from build123d import *

# Parameters (mm, degrees)
F1_DEPTH = 35.56
F2_W     = 27.6606
F2_H     = 23.5712
F4_DEPTH = 2.54
F7_DEPTH = 3.81
F8_DEPTH = 3.81


with BuildPart() as f1:
    # F0 (on Top) → F1 (new body)
    with BuildSketch(Plane.XY):
        Polygon((0, 12.2589374599), (0, 12.1117923089), (0, -11.4594076911), (2.54, -11.4594076911), (2.54, 12.2589374599), align=None)
    extrude(amount=F1_DEPTH)


with BuildPart() as f1_1:
    # F3: moved
    add(f1.part.moved(Location((-0.1992022446, -0.1268434648, 0))))

    # F2 (on Top) → F4 (join)
    with BuildSketch(Plane.XY):
        with Locations((16.1710977554, 0.1993488441)):
            Rectangle(F2_W, F2_H)
    extrude(amount=F4_DEPTH)

    # F5 (on face) → F7 (join)
    with BuildSketch(Plane.XZ.offset(11.5862511559)):
        Polygon((30.0013977554, 2.54), (2.3407977554, 35.56), (2.3407977554, 2.54), align=None)
    extrude(amount=-F7_DEPTH)

    # F6 (on face) → F8 (join)
    with BuildSketch(Plane(origin=(0, 12.1320939951, 0), x_dir=(-1, 0, 0), z_dir=(0, 1, 0))):
        Polygon((-2.3407977554, 35.56), (-30.0013977554, 2.54), (-2.3407977554, 2.54), align=None)
    extrude(amount=-F8_DEPTH)


solid = f1_1.part
Could you check a few things on this model? Use its own coordinates, in mm. A direction names the side the tool comes from. Coordinates: 2 decimals unless noted, no trailing zeros. Loops run counter-clockwise (first coordinate to the right, second up) from the corner with the lowest first, then second, coordinate; pieces in that order, holes last. Notation, with made-up numbers: (66, 35) -> (76, 35) arc R13 ccw to (76, 50) -> close; hole circle Ø6 at (0.5, 48). An arc over 180 degrees is marked (long way). Answer in a Markdown table with one row per item.
(1) Thinking about a two-plate mould opening in Y: for faces 4 (the face through (1, 0, 35.56)), 5 (the face through (8, 12.132, 14)), 6 (the face through (2.341, 0, 19)), which applies, released by +Y, released by -Y, zero draft, split by the parting line, or undercut?
Results found:
| item | result |
|---|---|
| face 4 | zero draft |
| face 5 | released by +Y |
| face 6 | undercut |
(2) For faces 1 (the face through (16, 0, 2.54)), 2 (the face through (16, 11.985, 1)), 3 (the face through (15, 0, 0)), which set-ups out of +Z, -Z, +X, -X, +Y, -Y let a thin tool reach every point of the face, with its end or its side?
Results found:
| item | result |
|---|---|
| face 1 | +Z, +X |
| face 2 | -Z, +X, +Y |
| face 3 | -Z, +X, -X, +Y, -Y |
(3) Imagine slicing it at D-D (x = 12.5). List the corners of the cut face in (y, z) for me.
Results found:
| item | result |
|---|---|
| outline | (-11.59, 0) -> (11.98, 0) -> (11.98, 2.54) -> (12.13, 2.54) -> (12.13, 23.43) -> (8.32, 23.43) -> (8.32, 2.54) -> (-7.78, 2.54) -> (-7.78, 23.43) -> (-11.59, 23.43) -> close |
(4) Will these pins go through, and if not, where does the flat tip stop? pin 1 Ø2 at (x, y) = (10.5, -9) entering from +Z; pin 2 Ø8 at (x, z) = (10, 28.5) entering from -Y; pin 3 Ø5 at (y, z) = (0, 12) entering from +X; pin 4 Ø1.5 at (x, y) = (10, 5.5) entering from +Z.
Results found:
| item | result |
|---|---|
| pin 1 | stops at z = 27.01 |
| pin 2 | stops at y = -11.59 |
| pin 3 | stops at x = 2.34 |
| pin 4 | stops at z = 2.54 |
(5) If I drill on probe 1 along Y at (x, z) = (11, 21); probe 2 along Z at (x, y) = (25.5, 4.25); probe 3 along X at (y, z) = (-6.25, 26.5), over which ranges is the centre line in solid material (lowest first)?
Results found:
| item | result |
|---|---|
| probe 1 | y = -11.59 to -7.78, 8.32 to 12.13 |
| probe 2 | z = 0 to 2.54 |
| probe 3 | x = -0.2 to 2.34 |
(6) Imagine slicing it at A-A (y = 10.25). List the corners of the cut face in (x, z) for me.
Results found:
| item | result |
|---|---|
| outline | (-0.2, 0) -> (30, 0) -> (30, 2.54) -> (2.34, 35.56) -> (-0.2, 35.56) -> close |
(7) Imagine slicing it at B-B (x = 22). List the corners of the cut face in (y, z) for me.
Results found:
| item | result |
|---|---|
| outline | (-11.59, 0) -> (11.98, 0) -> (11.98, 2.54) -> (12.13, 2.54) -> (12.13, 12.09) -> (8.32, 12.09) -> (8.32, 2.54) -> (-7.78, 2.54) -> (-7.78, 12.09) -> (-11.59, 12.09) -> close |
(8) Imagine slicing it at C-C (z = 10). List the corners of the cut face in (x, y) for me.
Results found:
| item | result |
|---|---|
| outline | (-0.2, -11.59) -> (23.75, -11.59) -> (23.75, -7.78) -> (2.34, -7.78) -> (2.34, 8.32) -> (23.75, 8.32) -> (23.75, 12.13) -> (-0.2, 12.13) -> close |
